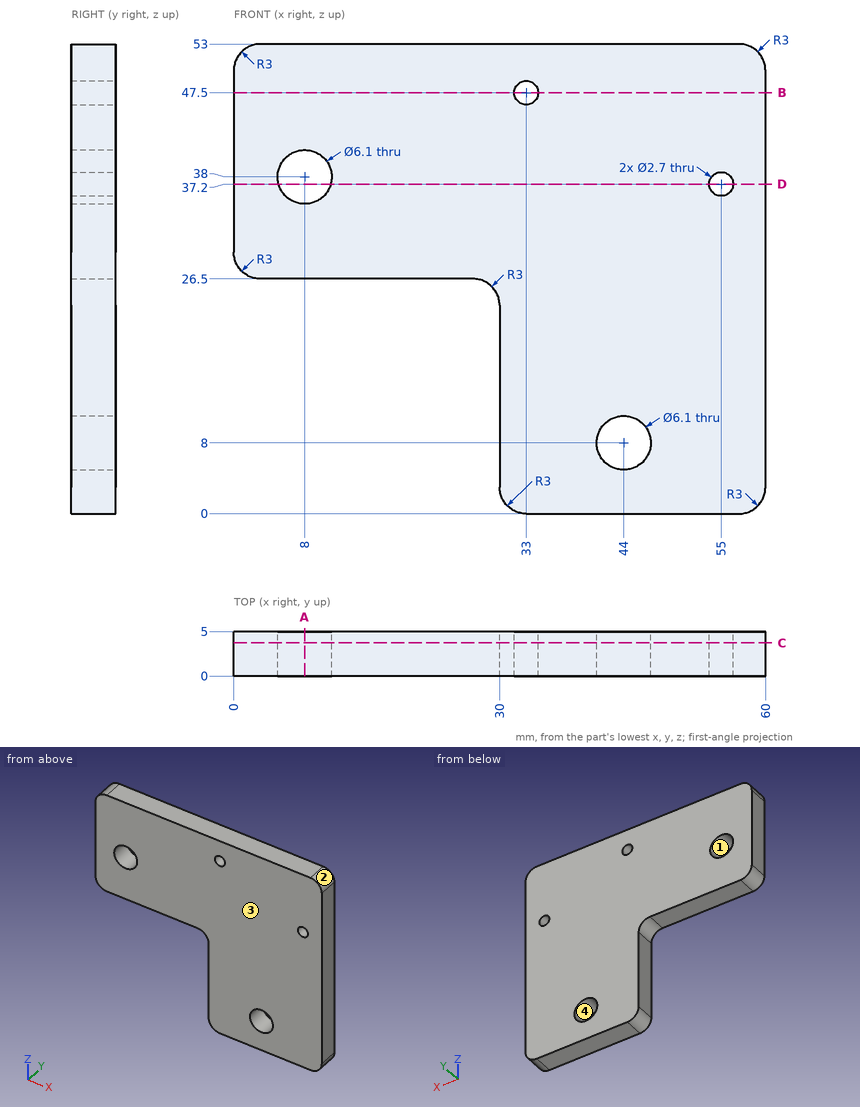
Geometry check sheet. Reference: drawing and pictorial views, mm from the part's lowest x, y, z. Coordinates: 2 decimals unless noted, no trailing zeros. Write each loop counter-clockwise with the first axis right and the second up, starting at its lowest first coordinate (ties: lowest second). Pieces come first, ordered by that corner, then holes.
Item 1: Cross-section at B-B on z = 47.5. Record the boundary of the cut face in (x, y).
Numbers:
outline: (0, 0) - (31.65, 0) - (31.65, 5) - (0, 5) - close; (34.35, 0) - (60, 0) - (60, 5) - (34.35, 5) - close
Item 2: Cross-section at C-C on y = 3.75. Record the boundary of the cut face in (x, z).
Numbers:
outline: (0, 29.5) arc R3 ccw to (3, 26.5) - (27, 26.5) arc R3 cw to (30, 23.5) - (30, 3) arc R3 ccw to (33, 0) - (57, 0) arc R3 ccw to (60, 3) - (60, 50) arc R3 ccw to (57, 53) - (3, 53) arc R3 ccw to (0, 50) - close; hole circle Ø6.1 at (8, 38); hole circle Ø2.7 at (33, 47.5); hole circle Ø6.1 at (44, 8); hole circle Ø2.7 at (55, 37.2)
Item 3: Depth check by flat-ended pin: pin 1 Ø1.5 at (y, z) = (3.5, 10) entering from -X; pin 2 Ø1 at (x, y) = (20.5, 2) entering from -Z. Enter the tip coordinate at first touch or a pass-through.
Numbers:
pin 1: stops at x = 30
pin 2: stops at z = 26.5
Item 4: Cross-section at A-A on x = 8. Record the boundary of the cut face in (y, z).
Numbers:
outline: (0, 26.5) - (5, 26.5) - (5, 34.95) - (0, 34.95) - close; (0, 41.05) - (5, 41.05) - (5, 53) - (0, 53) - close
Item 5: Mould release check, pull along X, two halves, no side actions. Record for the marked faces 1, 2, 3 and 4: released by +X, released by -X, zero draft, split by the parting line, or undercut.
Numbers:
face 1: undercut
face 2: released by +X
face 3: zero draft
face 4: undercut
Item 6: Cross-section at D-D on z = 37.2. Record the boundary of the cut face in (x, y), then the cut area to 3 significant figures.
Numbers:
outline: (0, 0) - (5.06, 0) - (5.06, 5) - (0, 5) - close; (10.94, 0) - (53.65, 0) - (53.65, 5) - (10.94, 5) - close; (56.35, 0) - (60, 0) - (60, 5) - (56.35, 5) - close
area: 257 mm2
Item 7: Scan lines: probe 1 along Z at (x, y) = (33, 2.8); probe 2 along X at (y, z) = (3.8, 38); probe 3 along Z at (x, y) = (44, 1.85). Record each from-to range of solid material in increasing order.
Numbers:
probe 1: z = 0 to 46.15, 48.85 to 53
probe 2: x = 0 to 4.95, 11.05 to 53.91, 56.09 to 60
probe 3: z = 0 to 4.95, 11.05 to 53
